Verification items for this drawing (mm, ordinates from the low corner). Round coordinates to 2 decimals unless told otherwise and drop trailing zeros. Loops run counter-clockwise (first coordinate to the right, second up) from the corner with the lowest first, then second, coordinate; pieces in that order, holes last. Notation, with made-up numbers: M -22,75 L -1,75 A29 cw -1,113 Z; hole C 33.25,36.5 d4. An arc over 180 degrees is marked long. Write item = value, one per line. Start each with the question number.
(1) Cross-section at B-B on x = 33. Record the boundary of the cut face in (y, z), plus the area to 3 significant figures.
(2) Cross-section at D-D on x = 43.5. Record the boundary of the cut face in (y, z).
(3) Scan lines: L1, parallel to X at y = 1.3, z = 3; L2, parallel to Z at x = 32, y = 1.8; L3, parallel to X at y = 1.3, z = 27.5. Record each from-to range of solid material in increasing order. Write a range as from..to.
(4) Go/stop test with flat-tipped pins: P1, Ø0.6, axis at x = 44, y = 1, coming from the -Z side; P2, Ø1, axis at y = 0.5, z = 32, coming from the +X side. Record where each tip stops, or that it passes through.
(5) Cross-section at C-C on y = 1.15. Record the boundary of the cut face in (x, z).
(6) Cross-section at A-A on z = 3. Record the boundary of the cut face in (x, y).
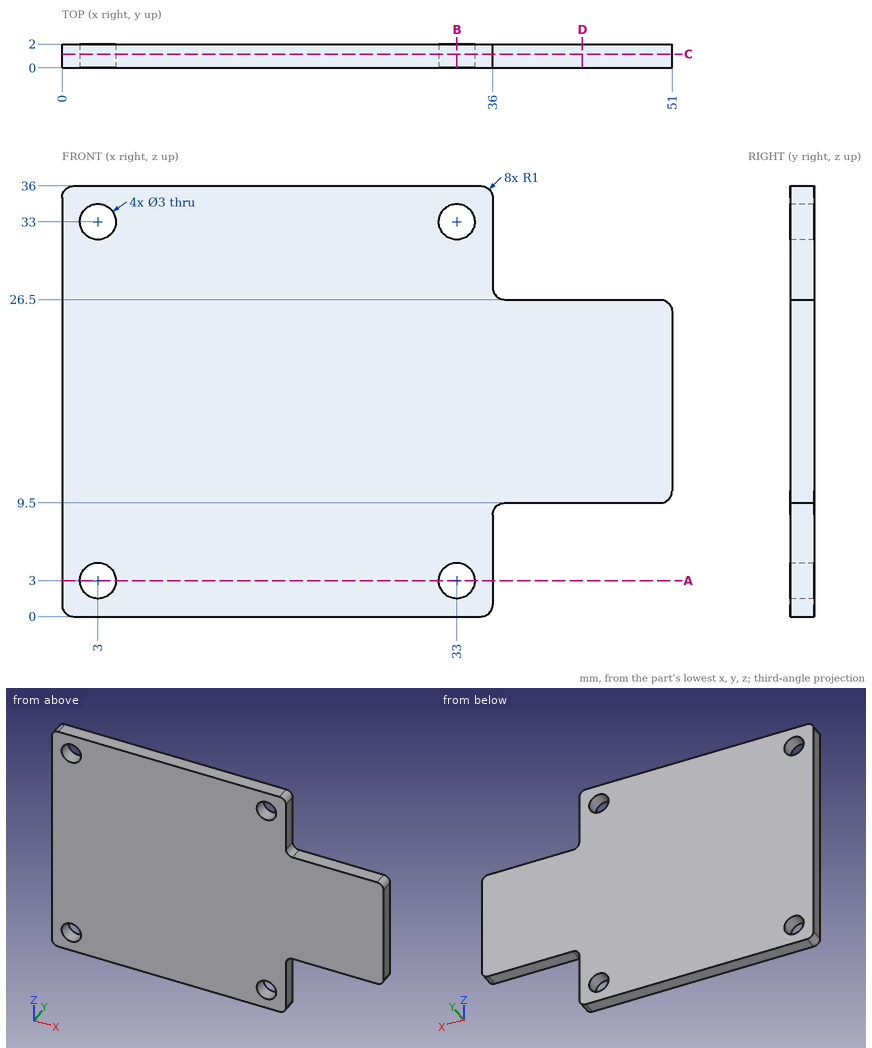
Result:
q1.outline = M 0,0 L 2,0 L 2,1.5 L 0,1.5 Z; M 0,4.5 L 2,4.5 L 2,31.5 L 0,31.5 Z; M 0,34.5 L 2,34.5 L 2,36 L 0,36 Z
q1.area = 60.0 mm^2
q2.outline = M 0,9.5 L 2,9.5 L 2,26.5 L 0,26.5 Z
q3.L1 = 0..1.5, 4.5..31.5, 34.5..36
q3.L2 = 0..1.88, 4.12..31.88, 34.12..36
q3.L3 = 0..36
q4.P1 = 9.5
q4.P2 = 36
q5.outline = M 0,1 A1 ccw 1,0 L 35,0 A1 ccw 36,1 L 36,8.5 A1 cw 37,9.5 L 50,9.5 A1 ccw 51,10.5 L 51,25.5 A1 ccw 50,26.5 L 37,26.5 A1 cw 36,27.5 L 36,35 A1 ccw 35,36 L 1,36 A1 ccw 0,35 Z; hole C 3,3 d3; hole C 3,33 d3; hole C 33,3 d3; hole C 33,33 d3
q6.outline = M 0,0 L 1.5,0 L 1.5,2 L 0,2 Z; M 4.5,0 L 31.5,0 L 31.5,2 L 4.5,2 Z; M 34.5,0 L 36,0 L 36,2 L 34.5,2 Z
